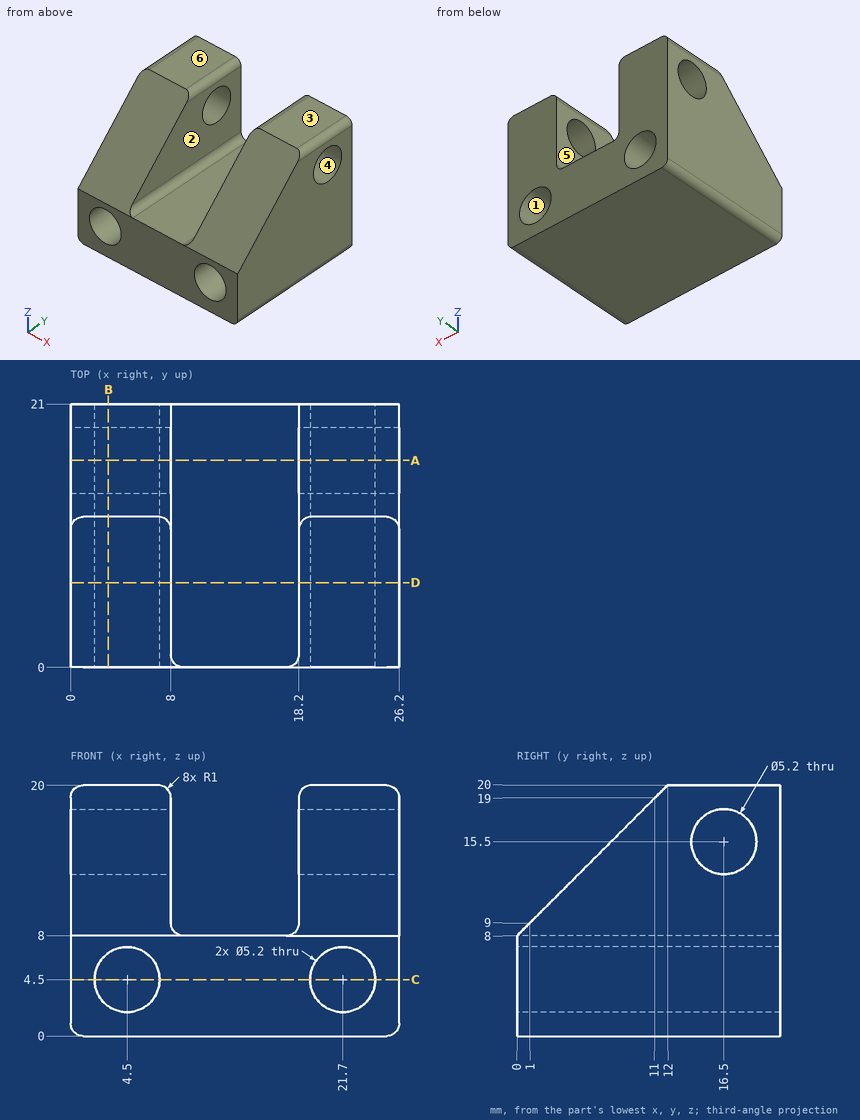
Design review of the part shown in the three views and the two pictorial views. Dimensions are in mm from the part's minimum x, y and z. A direction names the side the tool comes from. Round coordinates to 2 decimals unless told otherwise and drop trailing zeros. Write each loop counter-clockwise with the first axis right and the second up, starting at its lowest first coordinate (ties: lowest second). Pieces come first, ordered by that corner, then holes. Notation, with made-up numbers: M -15.5,69.25 L 41.5,69.25 A22 cw 41.5,88.25 Z; hole C 59.5,-7.75 d6. An arc over 180 degrees is marked long. One line per item, written item: value. Start each with the question number.
1. Draft analysis for pull direction Z (two halves, no side actions). For the marked faces 1, 2, 3 and 4, state which applies: pulls with the +Z half, pulls with the -Z half, needs draft (parallel to the pull), parting line crosses it, or undercut.
2. For the marked faces 5 and 6, list the 3-axis set-ups (+Z, -Z, +X, -X, +Y, -Y) from which the entire face can be reached by the end or side of a thin tool; tool diameter is ignored.
3. Clearance check with flat-ended pins moving along their axes: P1, Ø8, axis at x = 15.5, z = 14, coming from the -Y side; P2, Ø9, axis at x = 13.5, y = 12.5, coming from the +Z side. State where each tip first meets the part, or that it passes through.
4. To check wall thickness, follow probe 1 along X at (y, z) = (11.5, 4.5); probe 2 along X at (y, z) = (10.5, 14.25); probe 3 along X at (y, z) = (4.75, 5.25). State the ranges of each line that lie inside material, in increasing order. Write a range as from..to.
5. Take a section at A-A on y = 16.5. State the section outline as (x, z) points, then the cut area to 3 significant figures.
6. Take a section at D-D on y = 6.75. State the section outline as (x, z) points.
7. Take a section at C-C on z = 4.5. State the section outline as (x, y) points.
8. Take a section at B-B on x = 3. State the section outline as (y, z) points, then the cut area to 3 significant figures.
Computed:
1. face 1: undercut
1. face 2: needs draft
1. face 3: pulls with the +Z half
1. face 4: undercut
2. face 5: +Z, +Y, -Y
2. face 6: +Z, +X, -X, +Y, -Y
3. P1: stops at y = 3.05
3. P2: stops at z = 8.4
4. probe 1: x = 0..1.9, 7.1..19.1, 24.3..26.2
4. probe 2: x = 0..8, 18.2..26.2
4. probe 3: x = 0..2.01, 6.99..19.21, 24.19..26.2
5. outline: M 0,1 A1 ccw 1,0 L 25.2,0 A1 ccw 26.2,1 L 26.2,12.9 L 18.2,12.9 L 18.2,9 A1 cw 17.2,8 L 9,8 A1 cw 8,9 L 8,12.9 L 0,12.9 Z; M 0,18.1 L 8,18.1 L 8,19 A1 ccw 7,20 L 1,20 A1 ccw 0,19 Z; M 18.2,18.1 L 26.2,18.1 L 26.2,19 A1 ccw 25.2,20 L 19.2,20 A1 ccw 18.2,19 Z; hole C 4.5,4.5 d5.2; hole C 21.7,4.5 d5.2
5. area: 275 mm²
6. outline: M 0,1 A1 ccw 1,0 L 25.2,0 A1 ccw 26.2,1 L 26.2,14.75 L 18.2,14.75 L 18.2,9 A1 cw 17.2,8 L 9,8 A1 cw 8,9 L 8,14.75 L 0,14.75 Z; hole C 4.5,4.5 d5.2; hole C 21.7,4.5 d5.2
7. outline: M 0,0 L 1.9,0 L 1.9,21 L 0,21 Z; M 7.1,0 L 19.1,0 L 19.1,21 L 7.1,21 Z; M 24.3,0 L 26.2,0 L 26.2,21 L 24.3,21 Z
8. outline: M 0,0 L 21,0 L 21,2.38 L 0,2.38 Z; M 0,6.62 L 21,6.62 L 21,20 L 12,20 L 0,8 Z; hole C 16.5,15.5 d5.2
8. area: 238 mm²
